Part model, mm, in its own coordinate system. A direction names the side the tool comes from. Coordinates: 2 decimals unless noted, no trailing zeros. Loops run counter-clockwise (first coordinate to the right, second up) from the corner with the lowest first, then second, coordinate; pieces in that order, holes last. Notation, with made-up numbers: M 78,52 L 133,52 A21 cw 133,88 Z; hole C 81,52 d8. An arc over 180 degrees is marked long. Answer as a JSON object with one key per item and string values. Group by question number.
1. Saw through at A-A on y = -5. Write the cut outline in (x, z).
2. Mould opens along Y. For faces 1 (the face through (-0.01, 7.62, 9.37)), 2 (the face through (7.25, -2.35, 9.37)), 3 (the face through (4.424, -4.352, 9.367)) say: released by +Y, released by -Y, zero draft, split by the parting line, or undercut.
3. Saw through at C-C on x = 3.25. Write the cut outline in (y, z), then the cut area to 3 significant figures.
4. Saw through at D-D on y = 3.5. Write the cut outline in (x, z).
5. Saw through at B-B on x = -4.5. Write the cut outline in (y, z), then the cut area to 3 significant figures.
6. Drop flat-ended pins along their axis: pin 1 Ø4 at (x, z) = (-5, 7.5) entering from -Y; pin 2 Ø1 at (y, z) = (-5, 14) entering from +X; pin 3 Ø3 at (y, z) = (4.5, 11.5) entering from -X. Give the stop position or say it passes through.
7. Drill centre lines: L1, parallel to Y at x = 4.5, z = 5.25; L2, parallel to X at y = -5.25, z = 16; L3, parallel to Y at x = 4.25, z = 9. Where is each one in solid material? Low to high.
8. 3-axis set-ups, long thin cutter, end or side, ignore diameter. For faces 4 (the face through (-4.442, -4.39, 9.367)), 5 (the face through (4.442, 4.39, 9.367)), 6 (the face through (5.506, 2.862, 9.367)): which of +Z, -Z, +X, -X, +Y, -Y reach the whole face in a straight line?
Autodesk Inventor part; units mm, degrees
ref_plane "Work Plane2" through (0, 0, 9.5) normal (0, 0, 1) x (1, 0, 0)
ref_plane "Work Plane8" through (0, 0, 0) normal (0.9510565, 0.309017, 0) x (0, 0, 1)
ref_plane "Work Plane9" through (0, 0, 0) normal (1, 0, 0) x (0, 1, 0)
sketch "Sketch1" plane through (0, 0, 0) normal (0, 0, 1) x (1, 0, 0)
  circle A0 centre (0, 0) radius 7.62
  dimension "d0" = 15.24
extrude "Extrusion1" add sketch "Sketch1" along normal blind 19
ref_plane "Work Plane2" through (0, 0, 9.5) normal (0, 0, 1) x (1, 0, 0)
sketch "Sketch2" plane through (0, 0, 0) normal (0, 0, -1) x (-1, 0, 0)
  circle A0 centre (0, 0) radius 7.62
  circle A1 centre (0, 0) radius 6.35
  dimension "d3" = 12.7
surface extrude "Pitch Diameter" sketch "Sketch2" against normal through all shown no curves A1
ref_plane "Work Plane8" through (0, 0, 0) normal (0.9510565, 0.309017, 0) x (0, 0, 1)
ref_plane "Work Plane9" through (0, 0, 0) normal (1, 0, 0) x (0, 1, 0)
spur gear teeth "Spur Gear" teeth 10 pitch diameter 12.7 tip diameter 15.24 root diameter 9.525 face width 19 start plane through (0, 0, 0) normal (0, 0, -1) x (-1, 0, 0)
equation "\"d0\" = da_da"
equation "\"d1\" = da_b"
equation "\"d3\" = da_dw"
equation "\"d16\" = da_aw"
equation "\"d43\" = da_aw"
equation "\"d46\" = da_aw"
properties part number "Spur Gear1" material "Steel"
Outcome:
{
 "1": {"outline": "M -4.7,0 L -2.27,0 L -2.27,19 L -4.7,19 Z; M -1.12,0 L 1.12,0 L 1.12,19 L -1.12,19 Z; M 2.27,0 L 4.7,0 L 4.7,19 L 2.27,19 Z"},
 "2": {"face 1": "released by +Y", "face 2": "released by -Y", "face 3": "undercut"},
 "3": {"outline": "M -5.98,0 L 5.98,0 L 5.98,19 L -5.98,19 Z", "area": "227 mm²"},
 "4": {"outline": "M -3.92,0 L 3.92,0 L 3.92,19 L -3.92,19 Z"},
 "5": {"outline": "M -6.15,0 L -4.51,0 L -4.51,19 L -6.15,19 Z; M -2.64,0 L 2.64,0 L 2.64,19 L -2.64,19 Z; M 4.51,0 L 6.15,0 L 6.15,19 L 4.51,19 Z", "area": "162 mm²"},
 "6": {"pin 1": "stops at y = -6.5", "pin 2": "stops at x = 4.87", "pin 3": "stops at x = -4.95"},
 "7": {"L1": "y = -6.15 to -4.51, -2.64 to 2.64, 4.51 to 6.15", "L2": "x = -4.79 to -2.48, -1.11 to 1.11, 2.48 to 4.79", "L3": "y = -6.32 to -4.02, -2.56 to 2.56, 4.02 to 6.32"},
 "8": {"face 4": "+Z, -Z, -X", "face 5": "+Z, -Z, +X", "face 6": "+Z, -Z"}
}
